The model under review builds one solid part; all positions refer to its coordinate system, in mm. Face numbers are marked on the shaded views. A direction names the side the tool comes from. Coordinates: 2 decimals unless noted, no trailing zeros. Order: outer loops, then holes, each group sorted by start corner. A loop starts at its lowest first (then second) coordinate and runs counter-clockwise, first axis right, second up. Notation, with made-up numbers: (45, -35.75) -> (60, -35.75) arc R27 ccw to (60, 1.25) -> close; hole circle Ø9 at (-1.5, -36). An arc over 180 degrees is marked (long way). Put each result on its own line as item: value.
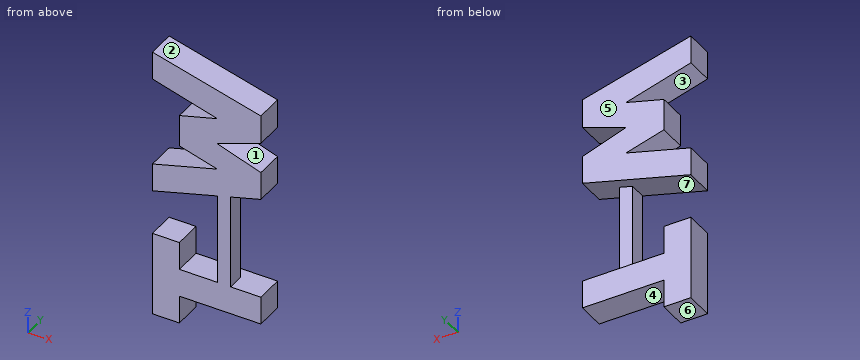
Autodesk Inventor part; units mm, degrees
ref_plane "YZ Plane" through (0, 0, 0) normal (1, 0, 0) x (0, 1, 0)
ref_plane "XZ Plane" through (0, 0, 0) normal (0, 1, 0) x (-1, 0, 0)
ref_plane "XY Plane" through (0, 0, 0) normal (0, 0, 1) x (1, 0, 0)
sketch "Sketch1" plane through (0, 0, 0) normal (0, 1, 0) x (-1, 0, 0)
  line L0 (6.2763, 15.9249) -> (6.2763, 10.9249)
  line L1 (6.2763, 10.9249) -> (-5.2771, 7.6502)
  line L2 (-5.2771, 7.6502) -> (1.4843, 5.8136)
  line L3 (1.4843, 5.8136) -> (1.4843, 0.1561)
  line L4 (1.4843, 0.1561) -> (-5.2771, -1.7603)
  line L5 (-5.2771, -1.7603) -> (6.2763, -4.934)
  line L6 (6.2763, -4.934) -> (6.2763, -9.934)
  line L7 (6.2763, -9.934) -> (-13.0093, -4.6363)
  line L8 (-13.0093, -4.6363) -> (-13.0093, 0.3637)
  line L9 (-13.0093, 0.3637) -> (-5.2771, 2.9849)
  line L10 (-5.2771, 2.9849) -> (-13.0093, 5.8136)
  line L11 (-13.0093, 5.8136) -> (-13.0093, 10.9249)
  line L12 (-13.0093, 10.9249) -> (6.2763, 15.9249)
  line L13 (6.2763, -17.865) -> (6.2763, -32.865)
  line L14 (6.2763, -32.865) -> (1.4843, -32.865)
  line L15 (1.4843, -32.865) -> (1.4843, -27.865)
  line L16 (1.4843, -27.865) -> (-13.0093, -27.865)
  line L17 (-13.0093, -27.865) -> (-13.0093, -22.865)
  line L18 (-13.0093, -22.865) -> (1.4843, -22.865)
  line L19 (1.4843, -22.865) -> (1.4843, -17.865)
  line L20 (1.4843, -17.865) -> (6.2763, -17.865)
  line L21 (-5.2771, -6.7603) -> (-5.2771, -22.865)
  line L22 (-7.6463, -22.865) -> (-7.6463, -6.1095)
  point P0 (0, 0)
extrude "Extrusion1" add sketch "Sketch1" along normal blind 5 contours L0 L1 L2 L3 L4 L5 L6 L7 L8 L9 L10 L11 L12 | L18 L19 L20 L13 L14 L15 L16 L17
extrude "Extrusion2" add sketch "Sketch1" along normal blind 3 contours L7 L21 L18 L22
properties part number "hw1-initials"
Item 1: For line 1 (Z direction, x = 2, y = 3.4) (3 decimals); line 2 (Z direction, x = 4.5, y = 1.15) (3 decimals); line 3 (X direction, y = 2, z = -18), list the stretches that pass through material, from the lowest coordinate up. Write a range as from..to.
Answers below:
line 1: -27.865..-22.865, -7.661..-2.661, -0.831..6.76, 8.579..13.779
line 2: -27.865..-22.865, -6.974..-1.974, -1.54..7.439, 7.87..13.131
line 3: -6.28..-1.48, 5.28..7.65
Item 2: For the marked faces 1, 2, 3 and 4, list the 3-axis set-ups (+Z, -Z, +X, -X, +Y, -Y) from which the entire face can be reached by the end or side of a thin tool; tool diameter is ignored.
Answers below:
face 1: +X, +Y, -Y
face 2: +Z, +X, +Y, -Y
face 3: -X, +Y, -Y
face 4: -Z, +X, +Y, -Y
Item 3: Consider section B-B on x = 4.25. Write out the cut boundary in (y, z) (3 decimals).
Answers below:
outline: (0, -27.865) -> (5, -27.865) -> (5, -22.865) -> (0, -22.865) -> close; (0, -7.042) -> (5, -7.042) -> (5, -2.042) -> (0, -2.042) -> close; (0, -1.469) -> (5, -1.469) -> (5, 7.371) -> (0, 7.371) -> close; (0, 7.941) -> (5, 7.941) -> (5, 13.196) -> (0, 13.196) -> close
Item 4: Consider section A-A on y = 4. Write out the cut boundary in (x, z) (3 decimals).
Answers below:
outline: (-6.276, -32.865) -> (-1.484, -32.865) -> (-1.484, -27.865) -> (13.009, -27.865) -> (13.009, -22.865) -> (-1.484, -22.865) -> (-1.484, -17.865) -> (-6.276, -17.865) -> close; (-6.276, -9.934) -> (13.009, -4.636) -> (13.009, 0.364) -> (5.277, 2.985) -> (13.009, 5.814) -> (13.009, 10.925) -> (-6.276, 15.925) -> (-6.276, 10.925) -> (5.277, 7.65) -> (-1.484, 5.814) -> (-1.484, 0.156) -> (5.277, -1.76) -> (-6.276, -4.934) -> close
Item 5: Consider section D-D on x = 6.5. Write out the cut boundary in (y, z) (1 decimal), and give its area (3 significant figures).
Answers below:
outline: (0, -27.9) -> (5, -27.9) -> (5, -22.9) -> (3, -22.9) -> (3, -6.4) -> (5, -6.4) -> (5, 2.6) -> (0, 2.6) -> close; (0, 3.4) -> (5, 3.4) -> (5, 12.6) -> (0, 12.6) -> close
area: 165 mm^2
Item 6: For pin 1 Ø1.5 at (y, z) = (1, -11) entering from +X; pin 2 Ø0.7 at (x, z) = (7, -15) entering from +Y; pin 3 Ø1 at (x, y) = (2, 1) entering from +Z, all flat-tipped, find the tip position at first contact; note any pin that passes through.
Answers below:
pin 1: x = 7.65
pin 2: y = 3
pin 3: z = 13.91
Item 7: Mouldability with a two-part tool opening along Z and no side actions: class the marked faces 5, 6 and 7 as +Z half, -Z half, draft (parallel to the pull), parting line (faces both ways), or undercut.
Answers below:
face 5: draft
face 6: -Z half
face 7: undercut
Item 8: Consider section C-C on z = -8. Write out the cut boundary in (x, y), and give its area (3 significant figures).
Answers below:
outline: (-6.28, 0) -> (0.76, 0) -> (0.76, 5) -> (-6.28, 5) -> close; (5.28, 0) -> (7.65, 0) -> (7.65, 3) -> (5.28, 3) -> close
area: 42.3 mm^2
